```python
from build123d import *

# Parameters (mm, degrees)
SKETCH_1_W          = 67
SKETCH_1_H          = 30
EXTRUDE_1_DEPTH     = 18.2
SKETCH_2_R          = 2
CUT_EXTRUDE_1_DEPTH = 19
SKETCH_3_W          = 10.5
SKETCH_3_H          = 30
CUT_EXTRUDE_2_DEPTH = 5


with BuildPart() as part:
    # 草图1 → 凸台-拉伸1 (new body)
    with BuildSketch(Plane.XY):
        Rectangle(SKETCH_1_W, SKETCH_1_H)
    extrude(amount=EXTRUDE_1_DEPTH)

    # 草图2 → 切除-拉伸1 (cut)
    with BuildSketch(Plane.XY.offset(18.2)):
        with Locations((-28.5, 0)):
            Circle(SKETCH_2_R)
        with Locations((28.5, 0)):
            Circle(SKETCH_2_R)
    extrude(amount=-CUT_EXTRUDE_1_DEPTH, mode=Mode.SUBTRACT)

    # 草图3 → 切除-拉伸2 (cut)
    with BuildSketch(Plane.XY.offset(18.2)):
        with Locations((-5.7, 0)):
            Rectangle(SKETCH_3_W, SKETCH_3_H)
        with Locations((-17.1, 0)):
            Rectangle(SKETCH_3_W, SKETCH_3_H)
        with Locations((17.1, 0)):
            Rectangle(SKETCH_3_W, SKETCH_3_H)
        with Locations((5.7, 0)):
            Rectangle(SKETCH_3_W, SKETCH_3_H)
    extrude(amount=-CUT_EXTRUDE_2_DEPTH, mode=Mode.SUBTRACT)


solid = part.part
```
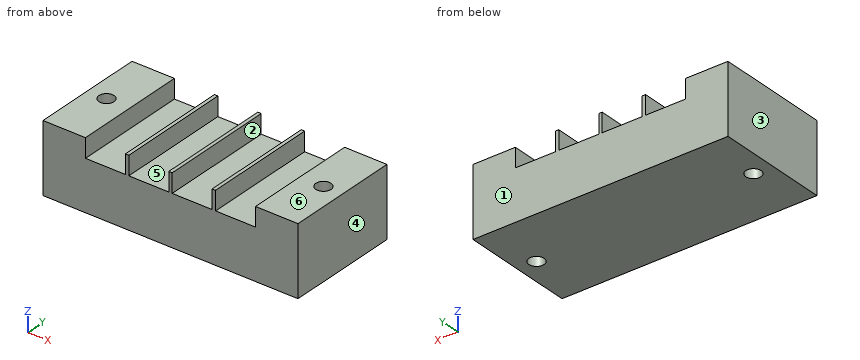
Verification items for the finished model (mm, model axes). Face numbers are marked on the shaded views. A direction names the side the tool comes from. Give positions to 0.01 mm unless a question says otherwise; leave off trailing zeros. Order: outer loops, then holes, each group sorted by start corner. A loop starts at its lowest first (then second) coordinate and runs counter-clockwise, first axis right, second up. Notation, with made-up numbers: M 72,24 L 101,24 A25 ccw 101,38 Z; hole C 4,-34 d11. An arc over 180 degrees is marked long. Return JSON: item names as keys, results as strings. Group by question number.
1) Scan lines: line 1 (X direction, y = 6.5, z = 13.25); line 2 (Y direction, x = -28.5, z = 9.75); line 3 (Z direction, x = 3, y = -9.75). Record each from-to range of solid material in increasing order.
2) Go/stop test with a flat-tipped pin: pin 1 Ø2 at (x, y) = (13, 2) entering from +Z. Record where the tip stops, or that it passes through.
3) Access from +Z, -Z, +X, -X, +Y, -Y to the whole of each face (thin tool, end or side, straight path). Record for the marked faces 5 and 6.
4) Section check C-C on y = 0. Record the cut outline in (x, z), and give its area (3 significant figures).
5) Mould release check, pull along X, two halves, no side actions. Record for the marked faces 1, 2, 3 and 4: pulls with the +X half, pulls with the -X half, needs draft (parallel to the pull), parting line crosses it, or undercut.
6) Section check D-D on y = -10.75. Record the cut outline in (x, z), and give its area (3 significant figures).
7) Section check A-A on x = 28.5. Record the cut outline in (y, z), and give its area (3 significant figures).
8) Section check B-B on z = 14.25. Record the cut outline in (x, y).
Answer block:
{
 "1": {"line 1": "x = -33.5 to -22.35, -11.85 to -10.95, -0.45 to 0.45, 10.95 to 11.85, 22.35 to 33.5", "line 2": "y = -15 to -2, 2 to 15", "line 3": "z = 0 to 13.2"},
 "2": {"pin 1": "stops at z = 13.2"},
 "3": {"face 5": "+Z, +Y, -Y", "face 6": "+Z, +X, -X, +Y, -Y"},
 "4": {"outline": "M -33.5,0 L -30.5,0 L -30.5,18.2 L -33.5,18.2 Z; M -26.5,0 L 26.5,0 L 26.5,18.2 L 22.35,18.2 L 22.35,13.2 L 11.85,13.2 L 11.85,18.2 L 10.95,18.2 L 10.95,13.2 L 0.45,13.2 L 0.45,18.2 L -0.45,18.2 L -0.45,13.2 L -10.95,13.2 L -10.95,18.2 L -11.85,18.2 L -11.85,13.2 L -22.35,13.2 L -22.35,18.2 L -26.5,18.2 Z; M 30.5,0 L 33.5,0 L 33.5,18.2 L 30.5,18.2 Z", "area": "864 mm^2"},
 "5": {"face 1": "needs draft", "face 2": "undercut", "face 3": "pulls with the -X half", "face 4": "pulls with the +X half"},
 "6": {"outline": "M -33.5,0 L 33.5,0 L 33.5,18.2 L 22.35,18.2 L 22.35,13.2 L 11.85,13.2 L 11.85,18.2 L 10.95,18.2 L 10.95,13.2 L 0.45,13.2 L 0.45,18.2 L -0.45,18.2 L -0.45,13.2 L -10.95,13.2 L -10.95,18.2 L -11.85,18.2 L -11.85,13.2 L -22.35,13.2 L -22.35,18.2 L -33.5,18.2 Z", "area": "1,010 mm^2"},
 "7": {"outline": "M -15,0 L -2,0 L -2,18.2 L -15,18.2 Z; M 2,0 L 15,0 L 15,18.2 L 2,18.2 Z", "area": "473 mm^2"},
 "8": {"outline": "M -33.5,-15 L -22.35,-15 L -22.35,15 L -33.5,15 Z; M -11.85,-15 L -10.95,-15 L -10.95,15 L -11.85,15 Z; M -0.45,-15 L 0.45,-15 L 0.45,15 L -0.45,15 Z; M 10.95,-15 L 11.85,-15 L 11.85,15 L 10.95,15 Z; M 22.35,-15 L 33.5,-15 L 33.5,15 L 22.35,15 Z; hole C -28.5,0 d4; hole C 28.5,0 d4"}
}
